Read the model definition and answer for the solid it produces. Units are mm, in the model's axes. A direction names the side the tool comes from. Coordinates: 2 decimals unless noted, no trailing zeros. Write each loop counter-clockwise with the first axis right and the second up, starting at its lowest first coordinate (ties: lowest second). Pieces come first, ordered by that corner, then holes. Notation, with made-up numbers: (24.25, 89) -> (81.25, 89) arc R26 ccw to (81.25, 121) -> close; hole circle Ø5 at (-33.5, 61). An arc over 180 degrees is marked (long way). Use CSV: the item, a comma, the result in double quotes.
from build123d import *

# Parameters (mm, degrees)
F0_R     = 2.5
F0_W     = 5
F0_H     = 80
F1_DEPTH = 5


with BuildPart() as f1:
    # F0 (on Top) → F1 (new body)
    with BuildSketch(Plane.XY):
        Polygon((30, -15), (30, 15), (-30, 15), (-30, -15), (-25, -15), (25, -15), align=None)
        with Locations((-20, 0)):
            Circle(F0_R, mode=Mode.SUBTRACT)
        with Locations((20, 0)):
            Circle(F0_R, mode=Mode.SUBTRACT)
        with Locations((27.5, -55)):
            Rectangle(F0_W, F0_H)
        with Locations((-27.5, -55)):
            Rectangle(F0_W, F0_H)
    extrude(amount=F1_DEPTH)


solid = f1.part
1. A cutting plane is placed at A-A (y = 0). Give the vertices of the cut face in (x, z).
Solutions:
outline,"(-30, 0) -> (-22.5, 0) -> (-22.5, 5) -> (-30, 5) -> close; (-17.5, 0) -> (17.5, 0) -> (17.5, 5) -> (-17.5, 5) -> close; (22.5, 0) -> (30, 0) -> (30, 5) -> (22.5, 5) -> close"
2. A cutting plane is placed at C-C (x = -20). Give the vertices of the cut face in (y, z), and give its area (3 significant figures).
Solutions:
outline,"(-15, 0) -> (-2.5, 0) -> (-2.5, 5) -> (-15, 5) -> close; (2.5, 0) -> (15, 0) -> (15, 5) -> (2.5, 5) -> close"
area,"125 mm^2"
3. For a pull along Y with two mould halves and no side action, classify faces 3 (the flat face through (30, -41, 2)), 4 (the cylindrical face through (-22.5, 0.1, 2.5)), 5 (the flat face through (0, -15, 2)) as pulls with the +Y half, pulls with the -Y half, needs draft (parallel to the pull), parting line crosses it, or undercut.
Solutions:
face 3,"needs draft"
face 4,"undercut"
face 5,"pulls with the -Y half"
4. A cutting plane is placed at D-D (y = -68). Give the vertices of the cut face in (x, z).
Solutions:
outline,"(-30, 0) -> (-25, 0) -> (-25, 5) -> (-30, 5) -> close; (25, 0) -> (30, 0) -> (30, 5) -> (25, 5) -> close"
5. Each of these flat-tipped pins is pushed along its axis until it touches: pin 1 Ø2.5 at (x, z) = (-10.5, 2) entering from -Y; pin 2 Ø3 at (x, y) = (20, 0) entering from +Z. Where does it stop, or does it pass through?
Solutions:
pin 1,"stops at y = -15"
pin 2,"passes through"
6. Find the intervals of material crossed by line 1 along Y through (x, z) = (20, 1.1); line 2 along X through (y, z) = (-54.5, 3.7); line 3 along Y through (x, z) = (-7, 2), in increasing order.
Solutions:
line 1,"y = -15 to -2.5, 2.5 to 15"
line 2,"x = -30 to -25, 25 to 30"
line 3,"y = -15 to 15"
7. A tool of negligible diameter and unlimited length cuts with its end or side. For faces 1 (the flat face through (-0.4, -14.8, 0)), 2 (the flat face through (-25, -56, 2)), from which of +Z, -Z, +X, -X, +Y, -Y can it reach the whole face along a straight path? Write none if from no direction.
Solutions:
face 1,"-Z, +X, -X, +Y, -Y"
face 2,"+Z, -Z, -Y"
8. A cutting plane is placed at B-B (z = 3.55). Give the vertices of the cut face in (x, y).
Solutions:
outline,"(-30, -95) -> (-25, -95) -> (-25, -15) -> (25, -15) -> (25, -95) -> (30, -95) -> (30, 15) -> (-30, 15) -> close; hole circle Ø5 at (-20, 0); hole circle Ø5 at (20, 0)"
